Could you check a few things on this model? Use its own coordinates, in mm. A direction names the side the tool comes from. Round coordinates to 2 decimals unless told otherwise and drop trailing zeros. Loops run counter-clockwise (first coordinate to the right, second up) from the corner with the lowest first, then second, coordinate; pieces in that order, holes last. Notation, with made-up numbers: (85, -7.5) -> (99, -7.5) arc R13 cw to (99, 5.5) -> close; hole circle Ø5 at (45.25, 70.25). An arc over 180 degrees is marked (long way). One line per item, written item: value.
from build123d import *


with BuildPart() as part:
    # Эскиз1 → Повернуть1 (revolve)
    with BuildSketch(Plane(origin=(0, 0, 0), x_dir=(1, 0, 0), z_dir=(0, 1, 0))):
        with BuildLine():
            Line((0, 0), (0, -32.749033403))
            Line((0, -32.749033403), (-0.579289322, -33.328322725))
            ThreePointArc((-0.579289322, -33.328322725), (-0.688268343, -33.35), (-0.75, -33.257612047))
            Line((-0.75, -33.257612047), (-0.75, -31.35))
            Line((-0.75, -31.35), (-0.495, -31.35))
            Line((-0.495, -31.35), (-0.495, -24.8))
            Line((-0.495, -24.8), (-0.68, -24.8))
            Line((-0.68, -24.8), (-0.68, -16.475))
            Line((-0.68, -16.475), (-0.579289322, -16.4))
            Line((-0.579289322, -16.4), (-0.68, -16.325))
            Line((-0.68, -16.325), (-0.68, -0.68))
            ThreePointArc((-0.68, -0.68), (-0.480832611, -0.199167389), (0, 0))
        make_face()
    revolve(axis=Axis((0, 0, 0), (0, 0, 1)))


solid = part.part
(1) For faces 1 (the face through (0.75, -0.03, 32.29)), 2 (the face through (-0.65, -0.2, 20.58)), which set-ups out of +Z, -Z, +X, -X, +Y, -Y let a thin tool reach every point of the face, with its end or its side?
Recorded:
face 1: +Z, -Z
face 2: -Z
(2) If I drill on L1, parallel to X at y = 0.05, z = 5; L2, parallel to Y at x = -0.1, z = 17.5; L3, parallel to X at y = -0.35, z = 22.5, over which ranges is the centre line in solid material (lowest first)?
Recorded:
L1: -0.68 to 0.68
L2: -0.67 to 0.67
L3: -0.58 to 0.58
(3) Thinking about a two-plate mould opening in Z: for faces 3 (the face through (0.107, 0.483, 28.029)), 4 (the face through (-0.65, -0.2, 8.39)), 5 (the face through (0.036, 0.161, 32.914)), which applies, released by +Z, released by -Z, zero draft, split by the parting line, or undercut?
Recorded:
face 3: undercut
face 4: zero draft
face 5: released by +Z
(4) If we section it at A-A, the plane z = 16: Please give me the cut outline in (x, y), then the cut area to 3 significant figures.
Recorded:
outline: circle Ø1.36 at (0, 0)
area: 1.45 mm²
